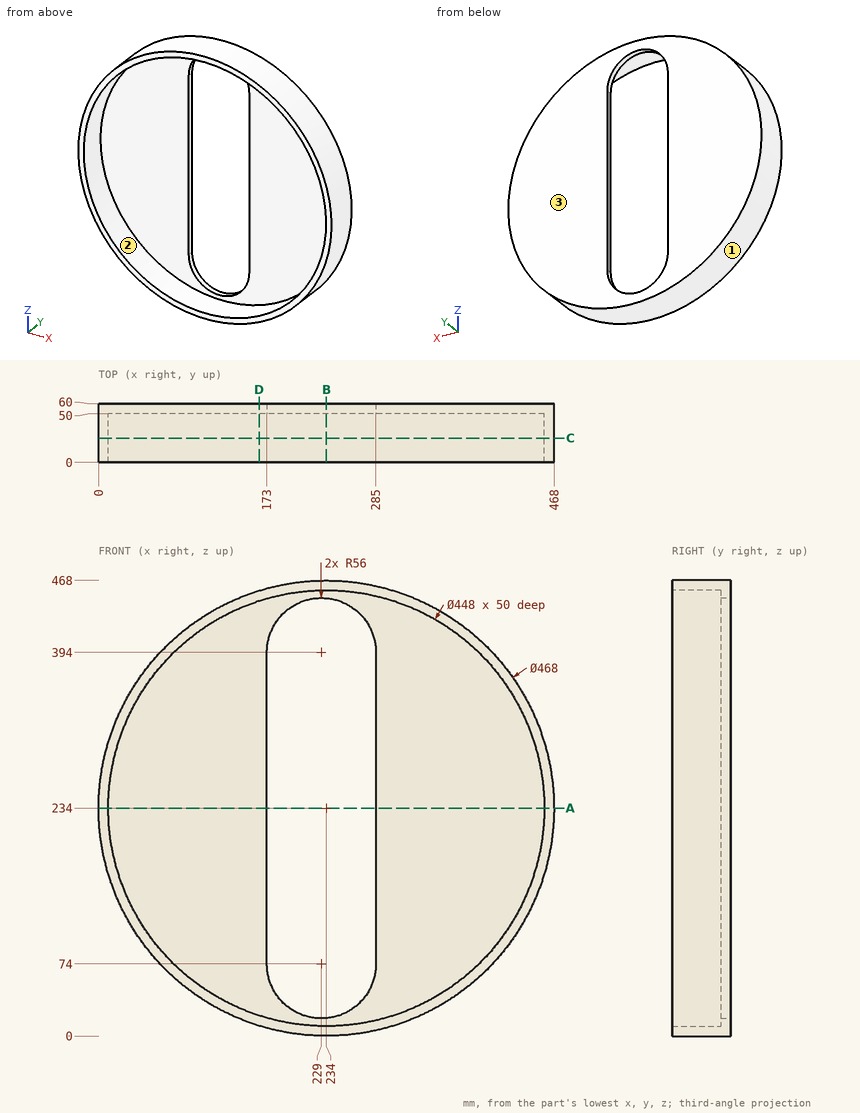
Could you check a few things on this drawing? It's one solid part, dimensions in mm from its lowest x, y, z. Give positions to 0.01 mm unless a question says otherwise; leave off trailing zeros. Write each loop counter-clockwise with the first axis right and the second up, starting at its lowest first coordinate (ties: lowest second). Pieces come first, ordered by that corner, then holes. Notation, with made-up numbers: (51, -10.5) - (67, -10.5) arc R32 ccw to (67, 17.5) - close; hole circle Ø10 at (18.25, 41). An arc over 180 degrees is marked (long way). Use CSV: the item, a comma, the result in double quotes. Start each with the question number.
Item 1: I want a section at A-A, the plane z = 234. Please give me the cut outline in (x, y), then the cut area to 3 significant figures.
Item 2: If we mould it in two halves opening along X, with no side actions, what happens to the marked faces 1, 2 and 3? For each: pulls with the +X half, pulls with the -X half, needs draft (parallel to the pull), parting line crosses it, or undercut.
Item 3: I want a section at B-B, the plane x = 234. Please give me the cut outline in (y, z), then the cut area to 3 significant figures.
Item 4: I'm going to push flat-ended pins straight in: pin 1 (3 mm diameter, centred on y = 57.5, z = 215.5, fed in from -X); pin 2 (8 mm diameter, centred on y = 31, z = 315, fed in from +X); pin 3 (10 mm diameter, centred on y = 41, z = 358, fed in from -X). Where does each tip first touch, or does it pass through?
Item 5: I want a section at D-D, the plane x = 165. Please give me the cut outline in (y, z), then the cut area to 3 significant figures.
Item 6: If I drill on line 1 along X through (y, z) = (24, 234); line 2 along Y through (x, z) = (95, 300); line 3 along Z through (x, y) = (269, 41), over which ranges is the centre line in solid material (lowest first)?
Item 7: I want a section at C-C, the plane y = 25. Please give me the cut outline in (x, z), then the cut area to 3 significant figures.
Findings:
1,outline,"(0, 0) - (10, 0) - (10, 50) - (173, 50) - (173, 60) - (0, 60) - close; (285, 50) - (458, 50) - (458, 0) - (468, 0) - (468, 60) - (285, 60) - close"
1,area,"4,560 mm2"
2,face 1,"parting line crosses it"
2,face 2,"undercut"
2,face 3,"needs draft"
3,outline,"(0, 0) - (60, 0) - (60, 18.22) - (50, 18.22) - (50, 10) - (0, 10) - close; (0, 458) - (50, 458) - (50, 449.78) - (60, 449.78) - (60, 468) - (0, 468) - close"
3,area,"1,360 mm2"
4,pin 1,"stops at x = 0.62"
4,pin 2,"stops at x = 454.97"
4,pin 3,"stops at x = 32.52"
5,outline,"(0, 10.4) - (60, 10.4) - (60, 457.6) - (0, 457.6) - (0, 447.11) - (50, 447.11) - (50, 20.89) - (0, 20.89) - close"
5,area,"5,520 mm2"
6,line 1,"x = 0 to 10, 458 to 468"
6,line 2,"y = 50 to 60"
6,line 3,"z = 2.63 to 12.75, 455.25 to 465.37"
7,outline,"circle Ø468 at (234, 234); hole circle Ø448 at (234, 234)"
7,area,"14,400 mm2"
